Autodesk Inventor part; units mm, degrees
ref_plane "YZ Plane" through (0, 0, 0) normal (1, 0, 0) x (0, 1, 0)
ref_plane "XZ Plane" through (0, 0, 0) normal (0, 1, 0) x (-1, 0, 0)
ref_plane "XY Plane" through (0, 0, 0) normal (0, 0, 1) x (1, 0, 0)
sketch "Sketch1" plane through (0, 0, 0) normal (0, 1, 0) x (-1, 0, 0)
  line L0 (10, 100) -> (-10, 100)
  line L1 (-10, 100) -> (-10, -100)
  line L2 (-10, -100) -> (10, -100)
  line L3 (10, -100) -> (10, 100)
  point P0 (0, 0)
  point P1 (10, 0)
  point P2 (0, 100)
  dimension "d0" = 20
  dimension "d1" = 200
extrude "Extrusion1" add sketch "Sketch1" along normal blind 5.334
sketch "Sketch2" plane through (-10, 0, 100) normal (0, 0, 1) x (1, 0, 0)
  line L0 (0, 5.334) -> (20, 5.334)
  line L1 (6, 5.334) -> (14, 5.334)
  line L2 (14, 5.334) -> (14, 0)
  line L3 (14, 0) -> (6, 0)
  line L4 (6, 0) -> (6, 5.334)
  line L5 (0, 0) -> (20, 0)
  point P0 (10, 0)
  point P1 (10, 0)
  dimension "d4" = 8
  dimension "d5" = 4
extrude "Extrusion2" add sketch "Sketch2" along normal blind 5.334
mirror "Mirror1" about plane through (0, 0, 0) normal (0, 0, 1) of "Extrusion2"
sketch "Sketch3" plane through (10, 0, 100) normal (1, 0, 0) x (0, 0, -1)
  line L0 (0, 5.334) -> (200, 5.334)
  line L1 (0, 0) -> (200, 0)
  line L2 (8, 5.334) -> (14, 5.334)
  line L3 (14, 5.334) -> (14, 0)
  line L4 (14, 0) -> (8, 0)
  line L5 (8, 0) -> (8, 5.334)
  line L6 (0, 0) -> (0, 5.334)
  point P0 (100, 0)
  dimension "d8" = 6
  dimension "d9" = 8
extrude "Extrusion3" cut sketch "Sketch3" against normal blind 5.334 contours L0 L3 L1 L5
pattern_linear "Rectangular Pattern1" count 3 spacing 25.4 along (0, 0, -1) of "Extrusion3"
mirror "Mirror2" about plane through (0, 0, 0) normal (0, 0, 1) of "Extrusion3", "Rectangular Pattern1"
mirror "Mirror3" about plane through (0, 0, 0) normal (1, 0, 0) of "Extrusion3", "Rectangular Pattern1", "Mirror2"
properties part number "base"
Read the model definition and answer for the solid it produces. Units are mm, in the model's axes. A direction names the side the tool comes from. Coordinates: 2 decimals unless noted, no trailing zeros. Order: outer loops, then holes, each group sorted by start corner. A loop starts at its lowest first (then second) coordinate and runs counter-clockwise, first axis right, second up. Notation, with made-up numbers: M 76.5,-10 L 87.5,-10 A22 ccw 87.5,24 Z; hole C -27.75,-15.5 d8. An arc over 180 degrees is marked long. Put each result on its own line as item: value. Start each with the question number.
Item 1: For faces 1 (the face through (-4, 3, -103)), 2 (the face through (7, 3, -66.6)), 3 (the face through (-4.666, 3, 89)), determine the directions among +Z, -Z, +X, -X, +Y, -Y from which every point of the face is accessible in a straight line to the end or side of a thin tool.
Item 2: Given pin 1 Ø1.6 at (y, z) = (2.5, 103) entering from -X; pin 2 Ø2.5 at (y, z) = (3.5, 101.5) entering from +X; pin 3 Ø2 at (x, z) = (-1.5, -29) entering from -Y; pin 4 Ø2.5 at (x, y) = (6.5, 3) entering from +Z, each flat-ended and moving along its own axis, determine where each tip first touches the part or whether it passes through.
Item 3: Section A-A, the plane z = 38.5 is taken. Determine the outline of the cut face in (x, y), plus the area to 3 significant figures.
Item 4: The mould has two halves that part along Z. Classify faces 4 (the face through (-7, 3, -60.6)), 5 (the face through (0, 3, -105.334)), 6 (the face through (-7, 3, -66.6)), 7 (the face through (0, 3, 105.334)): +Z half, -Z half, draft (parallel to the pull), parting line (faces both ways), or undercut.
Item 5: Consider probe 1 along Z at (x, y) = (-4.25, 3.65). Determine where the line is inside the solid, lowest interval first. Write a range as [from, to].
Computed:
1. face 1: -Z, -X, +Y, -Y
1. face 2: +X, +Y, -Y
1. face 3: -X, +Y, -Y
2. pin 1: stops at x = -4
2. pin 2: stops at x = 4
2. pin 3: stops at y = 0
2. pin 4: stops at z = 100
3. outline: M -4.67,0 L 4.67,0 L 4.67,5.33 L -4.67,5.33 Z
3. area: 49.8 mm2
4. face 4: undercut
4. face 5: -Z half
4. face 6: undercut
4. face 7: +Z half
5. probe 1: z = [-100, 100]
